```python
from build123d import *

# Parameters (mm, degrees)
SKETCH_C02_1_R   = 2.5
SKETCH_C02_1_R_2 = 6.85
EXTRUDE1_DEPTH   = 100


with BuildPart() as part:
    # Sketch C02-1 → Extrude1 (new body)
    with BuildSketch(Plane.XY):
        Polygon((-4, 20), (4, 20), (20, 20), (20, 4), (16, 4), (16, 7.2), (18.1, 7.2), (18.1, 11), (13.12132, 11), (10, 7.87868), (10, -7.87868), (13.12132, -11), (18.1, -11), (18.1, -7.2), (16, -7.2), (16, -4), (20, -4), (20, -20), (4, -20), (4, -16), (7.2, -16), (7.2, -18.1), (11, -18.1), (11, -13.12132), (7.87868, -10), (-7.87868, -10), (-11, -13.12132), (-11, -18.1), (-7.2, -18.1), (-7.2, -16), (-4, -16), (-4, -20), (-20, -20), (-20, -4), (-16, -4), (-16, -7.2), (-18.1, -7.2), (-18.1, -11), (-13.12132, -11), (-10, -7.87868), (-10, 7.87868), (-13.12132, 11), (-18.1, 11), (-18.1, 7.2), (-16, 7.2), (-16, 4), (-20, 4), (-20, 20), align=None)
        with Locations((-15.5, -15.5)):
            Circle(SKETCH_C02_1_R, mode=Mode.SUBTRACT)
        with Locations((-15.5, 15.5)):
            Circle(SKETCH_C02_1_R, mode=Mode.SUBTRACT)
        with Locations((15.5, -15.5)):
            Circle(SKETCH_C02_1_R, mode=Mode.SUBTRACT)
        with Locations((15.5, 15.5)):
            Circle(SKETCH_C02_1_R, mode=Mode.SUBTRACT)
        Circle(SKETCH_C02_1_R_2, mode=Mode.SUBTRACT)
        Polygon((-4, 18.1), (4, 18.1), (11, 18.1), (11, 13.12132), (7.87868, 10), (-7.87868, 10), (-11, 13.12132), (-11, 18.1), align=None, mode=Mode.SUBTRACT)
    extrude(amount=-EXTRUDE1_DEPTH)


solid = part.part
```
Input: part model. Units: mm. Frame: model coordinates. A direction names the side the tool comes from. Give positions to 0.01 mm unless a question says otherwise; leave off trailing zeros. Order: outer loops, then holes, each group sorted by start corner. A loop starts at its lowest first (then second) coordinate and runs counter-clockwise, first axis right, second up.
1. Mould query, pull axis X, two halves, no side actions, for faces 4 (the cylindrical face through (13, 15.6, -49.3)), 5 (the flat face through (20, 12, -49)), 6 (the flat face through (18, -4, -49)). Classes: released by +X, released by -X, zero draft, split by the parting line, or undercut.
Derived:
face 4: undercut
face 5: released by +X
face 6: zero draft
2. Section A-A on y = 0. Return the cut outline in (x, z).
Derived:
outline: (-10, -100) - (-6.85, -100) - (-6.85, 0) - (-10, 0) - close; (6.85, -100) - (10, -100) - (10, 0) - (6.85, 0) - close
3. Section B-B on y = -17. Return the cut outline in (x, z).
Derived:
outline: (-20, -100) - (-17.5, -100) - (-17.5, 0) - (-20, 0) - close; (-13.5, -100) - (-11, -100) - (-11, 0) - (-13.5, 0) - close; (-7.2, -100) - (-4, -100) - (-4, 0) - (-7.2, 0) - close; (4, -100) - (7.2, -100) - (7.2, 0) - (4, 0) - close; (11, -100) - (13.5, -100) - (13.5, 0) - (11, 0) - close; (17.5, -100) - (20, -100) - (20, 0) - (17.5, 0) - close
4. Section D-D on y = 15.5. Return the cut outline in (x, z), and give its area (3 significant figures).
Derived:
outline: (-20, -100) - (-18, -100) - (-18, 0) - (-20, 0) - close; (-13, -100) - (-11, -100) - (-11, 0) - (-13, 0) - close; (11, -100) - (13, -100) - (13, 0) - (11, 0) - close; (18, -100) - (20, -100) - (20, 0) - (18, 0) - close
area: 800 mm2
5. Section C-C on x = -2. Return the cut outline in (y, z), and give its area (3 significant figures).
Derived:
outline: (-10, -100) - (-6.55, -100) - (-6.55, 0) - (-10, 0) - close; (6.55, -100) - (10, -100) - (10, 0) - (6.55, 0) - close; (18.1, -100) - (20, -100) - (20, 0) - (18.1, 0) - close
area: 880 mm2
6. Reachability of faces 1 (the flat face through (-18, 4, -49)), 2 (the flat face through (0, 20, -49)), 3 (the flat face through (16, 6, -49)) from +Z, -Z, +X, -X, +Y, -Y: full face, straight path, thin tool, end or side. Return the list, or none.
Derived:
face 1: +Z, -Z, -X
face 2: +Z, -Z, +X, -X, +Y
face 3: +Z, -Z
7. Material intervals for L1, parallel to Y at x = -15.5, z = -70.5; L2, parallel to X at y = 7.5, z = -9; L3, parallel to Y at x = 0, z = -94, sorted ascending.
Derived:
L1: y = -20 to -18, -13 to -11, 11 to 13, 18 to 20
L2: x = -20 to -18.1, -10 to 10, 18.1 to 20
L3: y = -10 to -6.85, 6.85 to 10, 18.1 to 20
